Study the drawing (mm; zero at the part's minimum x, y, z) and answer. A direction names the side the tool comes from. Round coordinates to 2 decimals unless told otherwise and drop trailing zeros. Order: outer loops, then holes, each group sorted by start corner. A loop starts at its lowest first (then second) coordinate and runs counter-clockwise, first axis right, second up. Notation, with made-up numbers: (70.25, 0) - (123.25, 0) arc R28 ccw to (123.25, 31) - close; hole circle Ø2 at (78.25, -25). An arc over 180 degrees is marked (long way). Put each result on its own line as item: value. Start each with the question number.
Q1. Each of these flat-tipped pins is pushed along its axis until it touches: pin 1 Ø1.5 at (y, z) = (102.5, 3) entering from +X; pin 2 Ø4 at (y, z) = (17, 3) entering from -X; pin 3 Ø5 at (y, z) = (69, 21) entering from -X. Where does it stop, or does it pass through?
Q2. Which of the six approach directions +Z, -Z, +X, -X, +Y, -Y give full straight-line access (tool end or side, diameter ignored) to the marked faces 1, 2 and 3?
Q3. Section B-B on y = 77.5 is taken. Give the vertices of the cut face in (x, z).
Q4. Find the intervals of material crossed by line 1 along X through (y, z) = (108, 6); line 2 along X through (y, z) = (31.5, 3.5) (1 decimal); line 3 along Y through (x, z) = (10.5, 19.5) (1 decimal), in increasing order. Write a range as from..to.
Q5. Section C-C on x = 35 is taken. Give the vertices of the cut face in (y, z), then the cut area to 3 significant figures.
Q6. Section A-A on z = 16.5 is taken. Give the vertices of the cut face in (x, y), then the cut area to 3 significant figures.
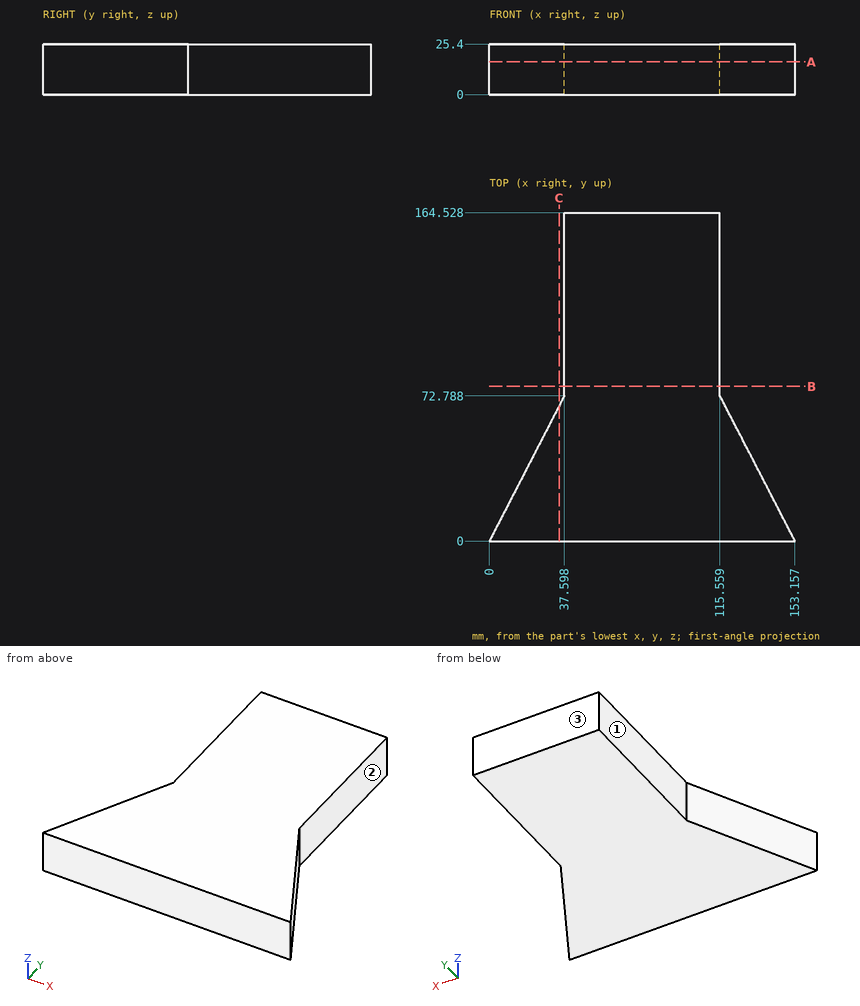
Findings:
1. pin 1: x = 115.56
1. pin 2: x = 7.75
1. pin 3: x = 34.35
2. face 1: +Z, -Z, -X, +Y
2. face 2: +Z, -Z, +X, +Y
2. face 3: +Z, -Z, +X, -X, +Y
3. outline: (37.6, 0) - (115.56, 0) - (115.56, 25.4) - (37.6, 25.4) - close
4. line 1: 37.6..115.56
4. line 2: 16.3..136.9
4. line 3: 0..20.3
5. outline: (0, 0) - (67.76, 0) - (67.76, 25.4) - (0, 25.4) - close
5. area: 1,720 mm2
6. outline: (0, 0) - (153.16, 0) - (115.56, 72.79) - (115.56, 164.53) - (37.6, 164.53) - (37.6, 72.79) - close
6. area: 15,600 mm2
